from build123d import *
from OCP.BRepFilletAPI import BRepFilletAPI_MakeChamfer

# Parameters (mm, degrees)
BOSS_EXTRUDE1_DEPTH = 6.35
CHAMFER1_SIZE       = 1.5875
CHAMFER1_SIZE2      = 2.749630657
CHAMFER2_SIZE       = 1.5875
CHAMFER2_SIZE2      = 2.749630657


with BuildPart() as part:
    # Sketch1 → Boss-Extrude1 (new body)
    with BuildSketch(Plane.XY):
        with BuildLine():
            Line((0, 0), (0, -63.5))
            ThreePointArc((0, -63.5), (12.7, -76.2), (25.4, -63.5))
            Line((25.4, -63.5), (25.4, 0))
            Line((25.4, 0), (0, 0))
        make_face()
    extrude(amount=BOSS_EXTRUDE1_DEPTH)

    # Chamfer1: one chamfer whose edges measure the first distance from different faces: ONE call of the kernel's chamfer builder (chamfer() names one face for all edges)
    chamfer1_edges_1 = [part.edges().sort_by_distance(p)[0] for p in [
        (12.7, -76.2, 6.35),
    ]]
    chamfer1_side_1 = [part.faces().sort_by_distance(p)[0] for p in [
        (12.7, -76.2, 3.175),
    ]]
    chamfer1_edges_2 = [part.edges().sort_by_distance(p)[0] for p in [
        (25.4, -31.75, 6.35),
    ]]
    chamfer1_side_2 = [part.faces().sort_by_distance(p)[0] for p in [
        (25.4, -31.75, 3.175),
    ]]
    chamfer1_edges_3 = [part.edges().sort_by_distance(p)[0] for p in [
        (0, -31.75, 6.35),
    ]]
    chamfer1_side_3 = [part.faces().sort_by_distance(p)[0] for p in [
        (0, -31.75, 3.175),
    ]]
    chamfer1 = BRepFilletAPI_MakeChamfer(part.part.solid().wrapped)
    for e in chamfer1_edges_1:
        chamfer1.Add(CHAMFER1_SIZE, CHAMFER1_SIZE2, e.wrapped, chamfer1_side_1[0].wrapped)  # the first distance lies on this face
    for e in chamfer1_edges_2:
        chamfer1.Add(CHAMFER1_SIZE, CHAMFER1_SIZE2, e.wrapped, chamfer1_side_2[0].wrapped)  # the first distance lies on this face
    for e in chamfer1_edges_3:
        chamfer1.Add(CHAMFER1_SIZE, CHAMFER1_SIZE2, e.wrapped, chamfer1_side_3[0].wrapped)  # the first distance lies on this face
    add(Compound.cast(chamfer1.Shape()), mode=Mode.REPLACE)

    # Chamfer2: one chamfer whose edges measure the first distance from different faces: ONE call of the kernel's chamfer builder (chamfer() names one face for all edges)
    chamfer2_edges_1 = [part.edges().sort_by_distance(p)[0] for p in [
        (25.4, -31.75, 0),
    ]]
    chamfer2_side_1 = [part.faces().sort_by_distance(p)[0] for p in [
        (25.4, -31.75, 2.38125),
    ]]
    chamfer2_edges_2 = [part.edges().sort_by_distance(p)[0] for p in [
        (12.7, -76.2, 0),
    ]]
    chamfer2_side_2 = [part.faces().sort_by_distance(p)[0] for p in [
        (12.7, -76.2, 2.38125),
    ]]
    chamfer2_edges_3 = [part.edges().sort_by_distance(p)[0] for p in [
        (0, -31.75, 0),
    ]]
    chamfer2_side_3 = [part.faces().sort_by_distance(p)[0] for p in [
        (0, -31.75, 2.38125),
    ]]
    chamfer2 = BRepFilletAPI_MakeChamfer(part.part.solid().wrapped)
    for e in chamfer2_edges_1:
        chamfer2.Add(CHAMFER2_SIZE, CHAMFER2_SIZE2, e.wrapped, chamfer2_side_1[0].wrapped)  # the first distance lies on this face
    for e in chamfer2_edges_2:
        chamfer2.Add(CHAMFER2_SIZE, CHAMFER2_SIZE2, e.wrapped, chamfer2_side_2[0].wrapped)  # the first distance lies on this face
    for e in chamfer2_edges_3:
        chamfer2.Add(CHAMFER2_SIZE, CHAMFER2_SIZE2, e.wrapped, chamfer2_side_3[0].wrapped)  # the first distance lies on this face
    add(Compound.cast(chamfer2.Shape()), mode=Mode.REPLACE)


solid = part.part
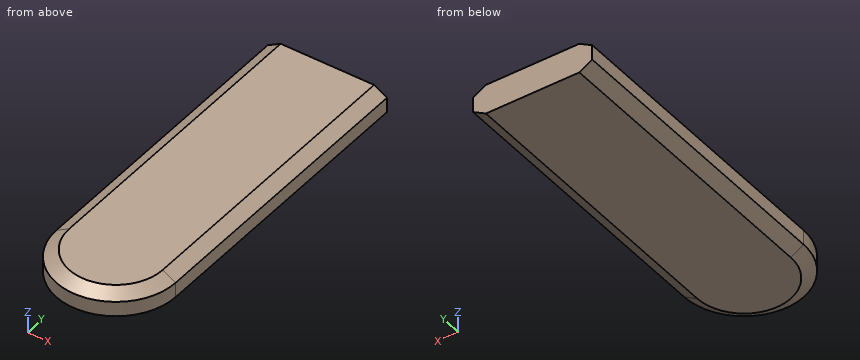
Design review of the part built by this model. Coordinates are the model's own, in mm. Round coordinates to 2 decimals unless told otherwise and drop trailing zeros. Loops run counter-clockwise (first coordinate to the right, second up) from the corner with the lowest first, then second, coordinate; pieces in that order, holes last. Notation, with made-up numbers: (52.5, -21) - (84.5, -21) arc R10 cw to (84.5, -12) - close; hole circle Ø6 at (-26.75, 5). An arc over 180 degrees is marked (long way). One line per question, with ' | ' between items.
1. We need section B-B, the plane z = 2.25. State the section outline as (x, y) points.
Results are:
outline: (0, -63.5) arc R12.7 ccw to (25.4, -63.5) - (25.4, 0) - (0, 0) - close
2. Clearance check with flat-ended pins moving along their axes: P1, Ø2, axis at x = 20, z = 1.5, coming from the +Y side; P2, Ø1, axis at y = -49.5, z = 1, coming from the +X side. State where each tip first meets the part, or that it passes through.
Results are:
P1: stops at y = 0 | P2: stops at x = 25.25
3. For L1, parallel to Z at x = 2.75, y = -64; L2, parallel to Y at x = 3.5, z = 4.5 (3 decimals); L3, parallel to Y at x = 10.75, z = 0.5, list the stretches that pass through material, from the lowest coordinate up. Write a range as [from, to].
Results are:
L1: z = [0.01, 6.34] | L2: y = [-72.255, 0] | L3: y = [-74.14, 0]
4. We need section A-A, the plane y = -56.5. State the section outline as (x, z) points.
Results are:
outline: (0, 1.59) - (2.75, 0) - (22.65, 0) - (25.4, 1.59) - (25.4, 4.76) - (22.65, 6.35) - (2.75, 6.35) - (0, 4.76) - close
